For this review, take the finished solid that the model builds, in its own axes (mm). Give positions to 0.01 mm unless a question says otherwise; leave off trailing zeros. Loops run counter-clockwise (first coordinate to the right, second up) from the corner with the lowest first, then second, coordinate; pieces in that order, holes last. Notation, with made-up numbers: (56, -39.75) - (68, -39.75) arc R26 ccw to (68, -12.75) - close; hole circle Ø2 at (35, -19). An arc over 180 degrees is marked (long way). Put each result on its own line as item: value.
from build123d import *

# Parameters (mm, degrees)
F1_DEPTH = 7.62


with BuildPart() as f1:
    # F0 (on Front) → F1 (new body)
    with BuildSketch(Plane.XZ):
        with BuildLine():
            Line((-3.8735, -29.845), (-3.8735, 0))
            Line((-3.8735, 0), (3.8735, 0))
            Line((3.8735, 0), (3.8735, -29.845))
            ThreePointArc((3.8735, -29.845), (4.431462, -31.192038), (5.7785, -31.75))
            Line((5.7785, -31.75), (6.4135, -31.75))
            ThreePointArc((6.4135, -31.75), (7.760538, -31.192038), (8.3185, -29.845))
            Line((8.3185, -29.845), (8.3185, -27.419537))
            ThreePointArc((8.3185, -27.419537), (9.468431, -19.863469), (12.814103, -12.991572))
            ThreePointArc((12.814103, -12.991572), (32.295171, 49.53), (12.814103, 112.051572))
            ThreePointArc((12.814103, 112.051572), (9.468431, 118.923469), (8.3185, 126.479537))
            Line((8.3185, 126.479537), (8.3185, 131.445))
            ThreePointArc((8.3185, 131.445), (7.760538, 132.792038), (6.4135, 133.35))
            Line((6.4135, 133.35), (5.7785, 133.35))
            ThreePointArc((5.7785, 133.35), (4.431462, 132.792038), (3.8735, 131.445))
            Line((3.8735, 131.445), (3.8735, 127))
            ThreePointArc((3.8735, 127), (0, 123.1265), (-3.8735, 127))
            Line((-3.8735, 127), (-3.8735, 131.445))
            ThreePointArc((-3.8735, 131.445), (-4.431462, 132.792038), (-5.7785, 133.35))
            Line((-5.7785, 133.35), (-6.4135, 133.35))
            ThreePointArc((-6.4135, 133.35), (-7.760538, 132.792038), (-8.3185, 131.445))
            Line((-8.3185, 131.445), (-8.3185, 126.479537))
            ThreePointArc((-8.3185, 126.479537), (-9.468431, 118.923469), (-12.814103, 112.051572))
            ThreePointArc((-12.814103, 112.051572), (-32.295171, 49.53), (-12.814103, -12.991572))
            ThreePointArc((-12.814103, -12.991572), (-9.468431, -19.863469), (-8.3185, -27.419537))
            Line((-8.3185, -27.419537), (-8.3185, -29.845))
            ThreePointArc((-8.3185, -29.845), (-7.760538, -31.192038), (-6.4135, -31.75))
            Line((-6.4135, -31.75), (-5.7785, -31.75))
            ThreePointArc((-5.7785, -31.75), (-4.431462, -31.192038), (-3.8735, -29.845))
        make_face()
        with BuildLine():
            ThreePointArc((-4.445, 18.441657), (-4.511776, 17.793916), (-4.709295, 17.173421))
            Line((-4.709295, 17.173421), (-8.054205, 9.496579))
            ThreePointArc((-8.054205, 9.496579), (-8.251724, 8.876084), (-8.3185, 8.228343))
            Line((-8.3185, 8.228343), (-8.3185, 2.670058))
            ThreePointArc((-8.3185, 2.670058), (-9.762051, 0.821791), (-11.904946, 1.774645))
            ThreePointArc((-11.904946, 1.774645), (-22.467997, 32.962926), (-22.501769, 65.891421))
            ThreePointArc((-22.501769, 65.891421), (-20.342296, 68.40201), (-17.123144, 67.625191))
            Line((-17.123144, 67.625191), (-5.374936, 55.876982))
            ThreePointArc((-5.374936, 55.876982), (-4.686682, 54.846938), (-4.445, 53.631918))
            Line((-4.445, 53.631918), (-4.445, 18.441657))
        make_face(mode=Mode.SUBTRACT)
        with BuildLine():
            ThreePointArc((8.3185, 8.20836), (8.247765, 8.874814), (8.038713, 9.511573))
            Line((8.038713, 9.511573), (4.724787, 16.873781))
            ThreePointArc((4.724787, 16.873781), (4.515735, 17.51054), (4.445, 18.176994))
            Line((4.445, 18.176994), (4.445, 38.391918))
            ThreePointArc((4.445, 38.391918), (6.40498, 41.325236), (9.865064, 40.636982))
            Line((9.865064, 40.636982), (20.466927, 30.035119))
            ThreePointArc((20.466927, 30.035119), (21.272034, 28.671577), (21.318445, 27.088767))
            ThreePointArc((21.318445, 27.088767), (17.456582, 14.11752), (11.904946, 1.774645))
            ThreePointArc((11.904946, 1.774645), (9.762051, 0.821791), (8.3185, 2.670058))
            Line((8.3185, 2.670058), (8.3185, 8.20836))
        make_face(mode=Mode.SUBTRACT)
        with BuildLine():
            ThreePointArc((-7.95743, 104.055176), (-5.817614, 104.861924), (-4.445, 103.032829))
            Line((-4.445, 103.032829), (-4.445, 68.898354))
            ThreePointArc((-4.445, 68.898354), (-6.40498, 65.965036), (-9.865064, 66.65329))
            Line((-9.865064, 66.65329), (-18.754319, 75.542545))
            ThreePointArc((-18.754319, 75.542545), (-19.587816, 77.011022), (-19.550592, 78.699145))
            ThreePointArc((-19.550592, 78.699145), (-14.627905, 91.776718), (-7.95743, 104.055176))
        make_face(mode=Mode.SUBTRACT)
        with BuildLine():
            ThreePointArc((4.445, 103.032829), (5.817614, 104.861924), (7.95743, 104.055176))
            ThreePointArc((7.95743, 104.055176), (20.919781, 73.664161), (23.445213, 40.720899))
            ThreePointArc((23.445213, 40.720899), (21.368761, 38.012906), (18.037106, 38.75112))
            Line((18.037106, 38.75112), (5.374936, 51.41329))
            ThreePointArc((5.374936, 51.41329), (4.686682, 52.443334), (4.445, 53.658354))
            Line((4.445, 53.658354), (4.445, 103.032829))
        make_face(mode=Mode.SUBTRACT)
    extrude(amount=F1_DEPTH)


solid = f1.part
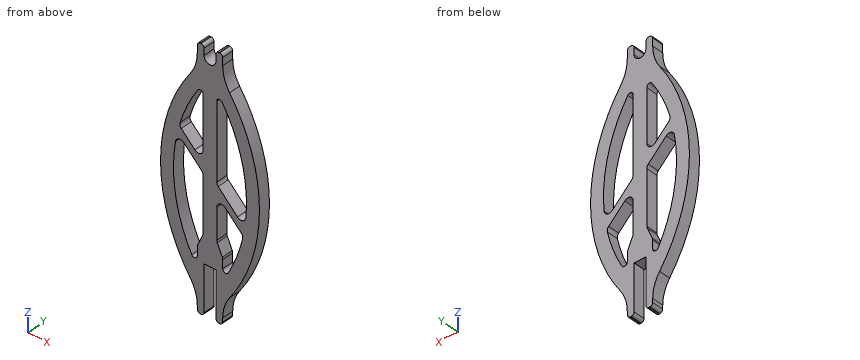
1) Insertion check: pin 1 Ø4 at (y, z) = (-3, 129) entering from -X; pin 2 Ø4 at (y, z) = (-3.5, 63.5) entering from -X; pin 3 Ø1.7 at (y, z) = (-5, 5.5) entering from +X. Each pin has a flat end and moves straight along its axis. Give the tip position at first contact, or say it passes through.
Geometry check:
pin 1: stops at x = -8.32
pin 2: stops at x = -31.64
pin 3: stops at x = 23.47
2) Take a section at C-C on x = 0. State the section outline as (y, z) points.
Geometry check:
outline: (-7.62, 0) - (0, 0) - (0, 123.13) - (-7.62, 123.13) - close
3) Take a section at A-A on y = -6. State how many separate pieces and enclosed holes the cut face has, and give its area (3 significant figures).
Geometry check:
separate pieces: 1
enclosed holes: 4
area: 4,240 mm²
4) Wall thickness on line 1 (Z direction, x = 12.5, y = -5.5); line 2 (Z direction, x = -14, y = -7); line 3 (X direction, y = -0.75, z = 69) (3 decimals): over which ranges is each line inside the solid? List them lowest first.
Geometry check:
line 1: z = -13.46 to 2.91, 38 to 44.29, 96.15 to 112.52
line 2: z = -11.24 to 5.94, 64.5 to 70.79, 93.12 to 110.3
line 3: x = -30.559 to -12.212, -4.445 to 4.445, 21.945 to 30.559
5) Take a section at B-B on x = -26. State the section outline as (y, z) points.
Geometry check:
outline: (-7.62, 12.84) - (0, 12.84) - (0, 86.22) - (-7.62, 86.22) - close
